from build123d import *

# Parameters (mm, degrees)
F0_W     = 16
F0_H     = 8
F0_W_2   = 9.43
F0_H_2   = 4.2
F1_DEPTH = 15
F2_W     = 16
F2_H     = 8
F3_DEPTH = 6
F4_R     = 3
F6_D     = 3
F7_R     = 1.5


with BuildPart() as f1:
    # F0 (on Top) → F1 (new body)
    with BuildSketch(Plane.XY):
        Rectangle(F0_W, F0_H)
        Rectangle(F0_W_2, F0_H_2, mode=Mode.SUBTRACT)
    extrude(amount=F1_DEPTH)

    # F2 (on face) → F3 (join)
    with BuildSketch(Plane.XZ.offset(4)):
        with Locations((0, 4)):
            Rectangle(F2_W, F2_H)
    extrude(amount=F3_DEPTH)

    # F4
    f4_edges = [f1.edges().sort_by_distance(p)[0] for p in [
        (0, -10, 0),
        (0, -10, 8),
    ]]
    fillet(f4_edges, radius=F4_R)

    # F6 (through all)
    with Locations(Plane(origin=(-8, 0, 0), x_dir=(0, -1, 0), z_dir=(-1, 0, 0))):
        with Locations((7, 4)):
            Hole(F6_D / 2)

    # F7
    f7_edges = [f1.edges().sort_by_distance(p)[0] for p in [
        (0, -4, 15),
        (0, 4, 15),
    ]]
    fillet(f7_edges, radius=F7_R)


solid = f1.part
Here's how the part is built. I have some questions about the finished solid (model axes, mm). A direction names the side the tool comes from. Coordinates: 2 decimals unless noted, no trailing zeros. Order: outer loops, then holes, each group sorted by start corner. A loop starts at its lowest first (then second) coordinate and runs counter-clockwise, first axis right, second up. Notation, with made-up numbers: (69, 62) -> (96, 62) arc R18 cw to (96, 90) -> close; hole circle Ø6 at (49.25, 53.5). An arc over 180 degrees is marked (long way). Answer in a Markdown table with one row per item.
(1) I want a section at C-C on y = 0.5. List the corners of the cut face in (x, z) for me (3 decimals).
Answer key:
| item | result |
|---|---|
| outline | (-8, 0) -> (-4.715, 0) -> (-4.715, 15) -> (-8, 15) -> close; (4.715, 0) -> (8, 0) -> (8, 15) -> (4.715, 15) -> close |
(2) I want a section at A-A on z = 4. List the corners of the cut face in (x, y) for me (3 decimals).
Answer key:
| item | result |
|---|---|
| outline | (-8, -10) -> (8, -10) -> (8, -8.5) -> (-8, -8.5) -> close; (-8, -5.5) -> (8, -5.5) -> (8, 4) -> (-8, 4) -> close; hole (-4.715, -2.1) -> (4.715, -2.1) -> (4.715, 2.1) -> (-4.715, 2.1) -> close |
(3) On a 3-axis mill with a long thin cutter (end or side, diameter ignored), from which of +Z, -Z, +X, -X, +Y, -Y can I reach the whole of each face in a straight line? I mean faces 4 (the face through (-4.715, 0, 7)), 5 (the face through (0, -5, 8)), 6 (the face through (0.11, -9.1, 0.86)). Say none if no direction works.
Answer key:
| item | result |
|---|---|
| face 4 | +Z, -Z |
| face 5 | +Z, +X, -X, -Y |
| face 6 | -Z, +X, -X, -Y |
(4) Thinking about a two-plate mould opening in Y: for faces 1 (the face through (-0.1, 2.3, 15)), 2 (the face through (4.715, 0, 7)), 3 (the face through (0.11, 3.57, 14.55)), which applies, +Y half, -Y half, draft (parallel to the pull), parting line (faces both ways), or undercut?
Answer key:
| item | result |
|---|---|
| face 1 | draft |
| face 2 | undercut |
| face 3 | +Y half |
(5) I want a section at B-B on x = -1.25. List the corners of the cut face in (y, z) for me.
Answer key:
| item | result |
|---|---|
| outline | (-10, 3) arc R3 ccw to (-7, 0) -> (-2.1, 0) -> (-2.1, 15) -> (-2.5, 15) arc R1.5 ccw to (-4, 13.5) -> (-4, 8) -> (-7, 8) arc R3 ccw to (-10, 5) -> close; (2.1, 0) -> (4, 0) -> (4, 13.5) arc R1.5 ccw to (2.5, 15) -> (2.1, 15) -> close; hole circle Ø3 at (-7, 4) |
(6) Please list where these lines run through material, in increasing order: probe 1 along Y at (x, z) = (-1.5, 13.5); probe 2 along Z at (x, y) = (4, -7); probe 3 along X at (y, z) = (0.75, 2) (3 decimals).
Answer key:
| item | result |
|---|---|
| probe 1 | -4 to -2.1, 2.1 to 4 |
| probe 2 | 0 to 2.5, 5.5 to 8 |
| probe 3 | -8 to -4.715, 4.715 to 8 |
(7) Will these pins go through, and if not, where does the flat tip stop? pin 1 Ø1 at (x, z) = (0, 8) entering from -Y; pin 2 Ø2.5 at (y, z) = (-7, 4) entering from +X; pin 3 Ø3.5 at (x, y) = (-3.5, -6) entering from +Z; pin 4 Ø4.5 at (x, z) = (-2, 11.5) entering from -Y.
Answer key:
| item | result |
|---|---|
| pin 1 | y = -8.66 |
| pin 2 | through |
| pin 3 | z = 8 |
| pin 4 | y = -4 |
(8) I want a section at D-D on x = -5.75. List the corners of the cut face in (y, z) for me, then the cut area to 3 significant figures.
Answer key:
| item | result |
|---|---|
| outline | (-10, 3) arc R3 ccw to (-7, 0) -> (4, 0) -> (4, 13.5) arc R1.5 ccw to (2.5, 15) -> (-2.5, 15) arc R1.5 ccw to (-4, 13.5) -> (-4, 8) -> (-7, 8) arc R3 ccw to (-10, 5) -> close; hole circle Ø3 at (-7, 4) |
| area | 156 mm^2 |
